Part model, mm, in its own coordinate system. A direction names the side the tool comes from. Coordinates: 2 decimals unless noted, no trailing zeros. Loops run counter-clockwise (first coordinate to the right, second up) from the corner with the lowest first, then second, coordinate; pieces in that order, holes last. Notation, with made-up numbers: M -13.75,5.25 L -8.75,5.25 A22 cw -8.75,11.25 Z; hole C -39.5,47 d3. An arc over 180 degrees is marked long. Use CSV: the item, a comma, the result in double quotes. Start each with the question number.
from build123d import *

# Parameters (mm, degrees)
F0_W          = 38
F0_H          = 20
F1_DEPTH      = 2
F2_R          = 2
F3_R          = 8
F4_DEPTH      = 2
F6_DEPTH      = 4
F6_DEPTH_BACK = 4


with BuildPart() as f1:
    # F0 (on Front) → F1 (new body)
    with BuildSketch(Plane.XZ):
        with BuildLine():
            add(Edge.make_bspline(
                [(19, -10), (14.1880401769, -12.4002225701), (11.0551596639, -15.0185183176), (8.6638560302, -19.389195231), (8, -22)],
                knots=[0, 0, 0, 0, 0.5443359888, 1, 1, 1, 1], degree=3))
            Line((19, -10), (-19, -10))
            add(Edge.make_bspline(
                [(-19, -10), (-14.1880401769, -12.4002225701), (-11.0551596639, -15.0185183176), (-8.6638560302, -19.389195231), (-8, -22)],
                knots=[0, 0, 0, 0, 0.5443359888, 1, 1, 1, 1], degree=3))
            Line((-8, -22), (0, -22))
            Line((0, -22), (8, -22))
        make_face()
        Rectangle(F0_W, F0_H)
    extrude(amount=F1_DEPTH)

    # F2
    f2_edges = [f1.edges().sort_by_distance(p)[0] for p in [
        (-19, -1, 10),
        (19, -1, 10),
        (-8, -1, -22),
        (8, -1, -22),
        (-19, -1, -10),
        (19, -1, -10),
    ]]
    fillet(f2_edges, radius=F2_R)

    # F3 (on face) → F4 (cut, through all)
    with BuildSketch(Plane.XZ.offset(2)):
        Circle(F3_R)
    extrude(amount=-F4_DEPTH, mode=Mode.SUBTRACT)

    # F5 (on Top) → F6 (join, two sides)
    with BuildSketch(Plane.XY) as f6_sk:
        Polygon((-19, 4), (-19, 0), (-17, 0), (-17, 2.2302730472), (-15.2302730472, 2.2302730472), (-17, 4), align=None)
        Polygon((17, 0), (19, 0), (19, 4), (17, 4), (15.2302730472, 2.2302730472), (17, 2.2302730472), align=None)
    extrude(amount=F6_DEPTH)
    extrude(f6_sk.sketch, amount=-F6_DEPTH_BACK)


solid = f1.part
1. Slice it at B-B, the plane x = 0. List the corners of the cut face in (y, z).
2. Wall check: probe 1 along Y at (x, z) = (13, 1.5); probe 2 along Z at (x, y) = (0, -1.3); probe 3 along Z at (x, y) = (1, -1.5). Give the ranges that are in metal, low to high.
3. Slice it at C-C, the plane y = 0.5. List the corners of the cut face in (x, z).
4. Slice it at A-A, the plane z = 0. List the corners of the cut face in (x, y).
5. Pin check, flat tips, straight feed: pin 1 (9.5 mm diameter, centred on x = 7, z = -2.5, fed in from +Y); pin 2 (2 mm diameter, centred on y = -0.5, z = -18.5, fed in from -X); pin 3 (1.9 mm diameter, centred on x = -17.5, y = 1.5, fed in from -Z). Stop position of each tip, or through.
6. Tool access for faces 1 (the face through (16, 2.23, 0)), 2 (the face through (0, -2, -9)), 3 (the face through (16, 3, 0)), 4 (the face through (-18, 2, -4)), 5 (the face through (-18, 2, 4)): list every direction of +Z, -Z, +X, -X, +Y, -Y with a clear straight run to the whole face (end or side of a thin tool).
7. Two-plate mould, pull along Y, no slides. Class faces 6 (the face through (-19, 0, 0)), 7 (the face through (-17, 1, 0)), 8 (the face through (-16, 3, 0)): pulls with the +Y half, pulls with the -Y half, needs draft (parallel to the pull), parting line crosses it, or undercut.
Found:
1,outline,"M -2,-22 L 0,-22 L 0,-8 L -2,-8 Z; M -2,8 L 0,8 L 0,10 L -2,10 Z"
2,probe 1,"-2 to 0"
2,probe 2,"-22 to -8, 8 to 10"
2,probe 3,"-22 to -7.94, 7.94 to 10"
3,outline,"M -19,-4 L -17,-4 L -17,4 L -19,4 Z; M 17,-4 L 19,-4 L 19,4 L 17,4 Z"
4,outline,"M -19,-2 L -8,-2 L -8,0 L -17,0 L -17,2.23 L -15.23,2.23 L -17,4 L -19,4 Z; M 8,-2 L 19,-2 L 19,4 L 17,4 L 15.23,2.23 L 17,2.23 L 17,0 L 8,0 Z"
5,pin 1,"y = 0"
5,pin 2,"x = -9.83"
5,pin 3,"z = -4"
6,face 1,"+Z, -Z"
6,face 2,"+Z, -Z, +X, -X, -Y"
6,face 3,"+Z, -Z, +Y"
6,face 4,"-Z, +X, -X, +Y"
6,face 5,"+Z, +X, -X, +Y"
7,face 6,"needs draft"
7,face 7,"undercut"
7,face 8,"pulls with the +Y half"
